The model under review builds one solid part; all positions refer to its coordinate system, in mm. Face numbers are marked on the shaded views. A direction names the side the tool comes from. Give positions to 0.01 mm unless a question says otherwise; leave off trailing zeros. Order: outer loops, then holes, each group sorted by start corner. A loop starts at its lowest first (then second) coordinate and runs counter-clockwise, first axis right, second up. Notation, with made-up numbers: (-22.75, 72) -> (34.25, 72) arc R30 cw to (34.25, 104) -> close; hole circle Ø1 at (70, 5.5). An arc over 180 degrees is marked (long way). Answer as a JSON object with one key per item and string values. Group by question number.
from build123d import *

# Parameters (mm, degrees)
OUTER_FRAME_EXTRUDE_DEPTH      = 4
OUTER_FRAME_EXTRUDE_DEPTH_BACK = 2
OUTSIDE_FRAME_W                = 18.2
OUTSIDE_FRAME_H                = 18.2
OUTSIDE_FRAME_W_2              = 14.2
OUTSIDE_FRAME_H_2              = 14.2
HOTSWAP_BASE_W                 = 18.2
HOTSWAP_BASE_H                 = 11.5
HOTSWAP_BASE_BLOCK_DEPTH       = 5
CUT_EXTRUDE4_DEPTH             = 16.704139582
CUT_EXTRUDE4_DEPTH_BACK        = 16.704139582
SKETCH1_W                      = 2
SKETCH1_H                      = 6.7
CUT_EXTRUDE1_DEPTH             = 4
SWITCH_PIN_HOLES_R             = 2
SWITCH_PIN_HOLES_R_2           = 1.25
SWITCH_HOLES_DEPTH             = 4
CUT_EXTRUDE3_REACH             = 17.704
HOTSWAP_HOLES_R                = 1.6
CHAMFER1_SIZE                  = 2
CHAMFER2_SIZE                  = 4.5
CHAMFER2_SIZE2                 = 4.997756317
FILLET1_R                      = 0.35


with BuildPart() as part:
    # Outside Frame → Outer Frame Extrude (new, two sides: drawn at the far end of the back side and taken through both)
    with BuildSketch(Plane.XY.offset(-4).offset(-OUTER_FRAME_EXTRUDE_DEPTH_BACK)):
        Rectangle(OUTSIDE_FRAME_W, OUTSIDE_FRAME_H)
        Rectangle(OUTSIDE_FRAME_W_2, OUTSIDE_FRAME_H_2, mode=Mode.SUBTRACT)
    extrude(amount=OUTER_FRAME_EXTRUDE_DEPTH + OUTER_FRAME_EXTRUDE_DEPTH_BACK)

    # Hotswap Base → Hotswap Base Block (add)
    with BuildSketch(Plane.XY.offset(-4)):
        with Locations((0, -3.35)):
            Rectangle(HOTSWAP_BASE_W, HOTSWAP_BASE_H)
    extrude(amount=-HOTSWAP_BASE_BLOCK_DEPTH)

    # Sketch1 → Cut-Extrude4 (cut, two sides: drawn at the far end of the back side and taken through both)
    with BuildSketch(Plane(origin=(0, 0, 0), x_dir=(0, 0, -1), z_dir=(1, 0, 0)).offset(-CUT_EXTRUDE4_DEPTH_BACK)):
        with Locations((5, 5.75)):
            Rectangle(SKETCH1_W, SKETCH1_H)
    extrude(amount=CUT_EXTRUDE4_DEPTH + CUT_EXTRUDE4_DEPTH_BACK, mode=Mode.SUBTRACT)

    # Hotswap Well → Cut-Extrude1 (cut)
    with BuildSketch(Plane(origin=(0, 0, -6), x_dir=(-1, 0, 0), z_dir=(0, 0, -1))):
        with BuildLine():
            Line((-10, -1.1), (-2.355843798, -1.1))
            ThreePointArc((-2.355843798, -1.1), (-1.396424004, -2.19317122), (0, -2.6))
            Line((0, -2.6), (5, -2.6))
            Line((5, -2.6), (5, -3.35))
            Line((5, -3.35), (10, -3.35))
            Line((10, -3.35), (10, -6.9))
            Line((10, -6.9), (-6, -6.9))
            Line((-6, -6.9), (-6, -4.1))
            Line((-6, -4.1), (-10, -4.1))
            Line((-10, -4.1), (-10, -1.1))
        make_face()
    extrude(amount=CUT_EXTRUDE1_DEPTH, mode=Mode.SUBTRACT)

    # Switch Pin Holes → Switch Holes (cut)
    with BuildSketch(Plane.XY.offset(-4)):
        Circle(SWITCH_PIN_HOLES_R)
        with Locations((-5, 0)):
            Circle(SWITCH_PIN_HOLES_R_2)
        with Locations((5, 0)):
            Circle(SWITCH_PIN_HOLES_R_2)
    extrude(amount=-SWITCH_HOLES_DEPTH, mode=Mode.SUBTRACT)

    # Cut-Extrude3: up to this face of the body (flat: up to its plane)
    cut_extrude3_end = Plane(part.part.faces().sort_by_distance((5, 0.029137252, -8))[0])
    # Hotswap Holes → Cut-Extrude3 (cut, up to the picked face)
    with BuildSketch(Plane.XY, mode=Mode.PRIVATE) as cut_extrude3_sk1:
        with Locations((-2.560136595, -4.965291588)):
            Circle(HOTSWAP_HOLES_R)
    cut_extrude3_tool1 = split(extrude(cut_extrude3_sk1.sketch, amount=-CUT_EXTRUDE3_REACH, mode=Mode.PRIVATE), bisect_by=cut_extrude3_end, keep=Keep.BOTH, mode=Mode.PRIVATE)
    # Hotswap Holes → Cut-Extrude3 (cut, up to the picked face)
    with BuildSketch(Plane.XY, mode=Mode.PRIVATE) as cut_extrude3_sk2:
        with BuildLine():
            Line((3.930924016, 0.647747281), (2.46548889, -1.77088348))
            ThreePointArc((2.46548889, -1.77088348), (3.179147124, -4.059894044), (5.3631684, -3.070485887))
            Line((5.3631684, -3.070485887), (6.194736133, -0.367567099))
            ThreePointArc((6.194736133, -0.367567099), (5.511530489, 1.140542222), (3.930924016, 0.647747281))
        make_face()
    cut_extrude3_tool2 = split(extrude(cut_extrude3_sk2.sketch, amount=-CUT_EXTRUDE3_REACH, mode=Mode.PRIVATE), bisect_by=cut_extrude3_end, keep=Keep.BOTH, mode=Mode.PRIVATE)
    add(cut_extrude3_tool1.solids().sort_by(Axis((-2.560137, -4.965292, 0), (0, 0, -1)))[0], mode=Mode.SUBTRACT)
    add(cut_extrude3_tool2.solids().sort_by(Axis((4.301523, -1.557372, 0), (0, 0, -1)))[0], mode=Mode.SUBTRACT)

    # Chamfer1
    chamfer1_edges = [part.edges().sort_by_distance(p)[0] for p in [
        (9.1, -4.1, -7.5),
        (-9.1, -6.9, -7.5),
        (-9.1, -3.35, -7.5),
        (9.1, -1.1, -7.5),
    ]]
    chamfer(chamfer1_edges, length=CHAMFER1_SIZE)

    # Chamfer2
    chamfer2_edges = [part.edges().sort_by_distance(p)[0] for p in [
        (-8.1, 2.4, -4),
        (8.1, 2.4, -4),
    ]]
    chamfer2_side = [part.faces().sort_by_distance(p)[0] for p in [
        (8.1, 2.593940713, -4),
    ]]
    chamfer(chamfer2_edges, length=CHAMFER2_SIZE, length2=CHAMFER2_SIZE2, reference=chamfer2_side[0])

    # Fillet1
    fillet1_edges = [part.edges().sort_by_distance(p)[0] for p in [
        (6, -4.1, -7.5),
        (-5, -3.35, -7.5),
        (-5, -2.6, -7.5),
        (6, -6.9, -7.5),
        (2.355843798, -1.1, -7.5),
    ]]
    fillet(fillet1_edges, radius=FILLET1_R)

    # Split1
    split(bisect_by=Plane.XY.offset(-4), keep=Keep.BOTTOM)


solid = part.part
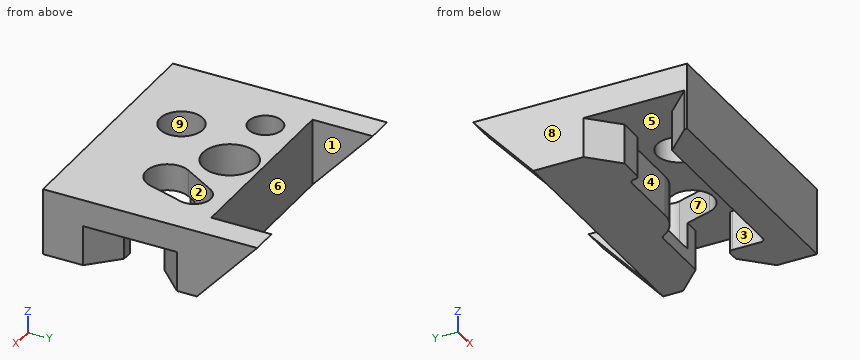
1. Take a section at B-B on x = -3.25. Give the boundary of the cut face in (y, z), plus the area to 3 significant figures.
2. Draft analysis for pull direction Y (two halves, no side actions). For the marked faces 6, 7, 8 and 9, state which applies: pulls with the +Y half, pulls with the -Y half, needs draft (parallel to the pull), parting line crosses it, or undercut.
3. Take a section at A-A on z = -7.4. State how many separate pieces and enclosed holes the cut face has, plus the area to 3 significant figures.
4. For probe 1 along Y at (x, z) = (0, -6.3); probe 2 along Y at (x, z) = (-2.75, -8.4); probe 3 along Y at (x, z) = (-2.5, -4.2), list the stretches that pass through material, from the lowest coordinate up. Write a range as [from, to].
5. For pin 1 (1.2 mm diameter, centred on x = -1, y = 0, fed in from +Z); pin 2 (1.5 mm diameter, centred on x = 2, z = -5.5, fed in from +Y); pin 3 (1.5 mm diameter, centred on y = 0, z = -7, fed in from +X); pin 4 (2.5 mm diameter, centred on x = 3.83, y = -2.6, fed in from -Z), all flat-tipped, find the tip position at first contact; note any pin that passes through.
6. Machinability: for the marked faces 1, 2, 3, 4 and 5, which of the approach directions +Z, -Z, +X, -X, +Y, -Y give a long, thin tool a straight path to every point of the face, cutting with its end or side? Answer none if there is none.
7. Take a section at D-D on x = -6. Give the boundary of the cut face in (y, z), plus the area to 4 significant figures.
8. Take a section at C-C on y = -5.5. Give the boundary of the cut face in (x, z).
Checks:
{
 "1": {"outline": "(-9.1, -9) -> (-6.9, -9) -> (-6.9, -6) -> (-6.41, -6) -> (-6.41, -4) -> (-9.1, -4) -> close; (-3.52, -6) -> (-2.6, -6) -> (-2.6, -9) -> (2.4, -9) -> (2.4, -4) -> (-3.52, -4) -> close", "area": "38.8 mm2"},
 "2": {"face 6": "pulls with the +Y half", "face 7": "undercut", "face 8": "needs draft", "face 9": "undercut"},
 "3": {"separate pieces": "2", "enclosed holes": "2", "area": "106 mm2"},
 "4": {"probe 1": "y = [-9.1, -6.9], [-2.6, -2], [2, 2.4]", "probe 2": "y = [-9.1, -6.9], [-2.6, 2.4]", "probe 3": "y = [-9.1, -6.56], [-3.37, 2.4]"},
 "5": {"pin 1": "stops at z = -8", "pin 2": "stops at y = 2.4", "pin 3": "stops at x = 8.95", "pin 4": "passes through"},
 "6": {"face 1": "+Z, -Z, +Y", "face 2": "+Z", "face 3": "-Z, -X", "face 4": "-Z, +X", "face 5": "-Z"},
 "7": {"outline": "(-9.1, -9) -> (-6.9, -9) -> (-6.9, -6) -> (-3.35, -6) -> (-3.35, -9) -> (2.4, -9) -> (2.4, -4) -> (0.75, -4) -> (0.75, -8) -> (-0.75, -8) -> (-0.75, -4) -> (-9.1, -4) -> close", "area": "40.85 mm2"},
 "8": {"outline": "(-9.1, -6) -> (-4.07, -6) -> (-4.07, -4) -> (-9.1, -4) -> close; (-1.05, -6) -> (6, -6) -> (6, -9) -> (8.5, -9) -> (8.5, -6) -> (9.1, -6) -> (9.1, -4) -> (-1.05, -4) -> close"}
}
